Geometry: final body of the model. Coordinates: model frame, mm. A direction names the side the tool comes from. Give positions to 0.01 mm unless a question says otherwise; leave off trailing zeros. Order: outer loops, then holes, each group sorted by start corner. A loop starts at its lowest first (then second) coordinate and runs counter-clockwise, first axis right, second up. Notation, with made-up numbers: (-17.5, -39) - (3.5, -39) arc R25 ccw to (3.5, -26) - close; hole circle Ø1 at (-6.5, -3). An arc over 180 degrees is marked (long way). Use one line per item in the form item = value.
from build123d import *

# Parameters (mm, degrees)
SKETCH_1_R          = 25
EXTRUDE_1_DEPTH     = 4
SKETCH_4_R          = 2.05
CUT_EXTRUDE_1_DEPTH = 10
SKETCH_5_R          = 4.05
SKETCH_5_R_2        = 2.05
CUT_EXTRUDE_2_DEPTH = 1
SKETCH_6_R          = 25
SKETCH_6_R_2        = 20
CUT_EXTRUDE_3_DEPTH = 0.5


with BuildPart() as part:
    # 草图1 → 凸台-拉伸1 (new body)
    with BuildSketch(Plane.XY):
        Circle(SKETCH_1_R)
    extrude(amount=EXTRUDE_1_DEPTH)

    # 草图4 → 切除-拉伸1 (cut)
    with BuildSketch(Plane(origin=(0, 0, 0), x_dir=(-1, 0, 0), z_dir=(0, 0, -1))):
        with Locations((-10.392304845, -6)):
            Circle(SKETCH_4_R)
        with Locations((-10.392304845, 6)):
            Circle(SKETCH_4_R)
        with Locations((0, 12)):
            Circle(SKETCH_4_R)
        with Locations((10.392304845, 6)):
            Circle(SKETCH_4_R)
        with Locations((10.392304845, -6)):
            Circle(SKETCH_4_R)
        with Locations((0, -12)):
            Circle(SKETCH_4_R)
    extrude(amount=-CUT_EXTRUDE_1_DEPTH, mode=Mode.SUBTRACT)

    # 草图5 → 切除-拉伸2 (cut)
    with BuildSketch(Plane.XY.offset(4)):
        with Locations((-10.392304845, 6)):
            Circle(SKETCH_5_R)
        with Locations((-10.392304845, 6)):
            Circle(SKETCH_5_R_2, mode=Mode.SUBTRACT)
        with Locations((-10.392304845, -6)):
            Circle(SKETCH_5_R)
        with Locations((-10.392304845, -6)):
            Circle(SKETCH_5_R_2, mode=Mode.SUBTRACT)
        with Locations((0, -12)):
            Circle(SKETCH_5_R)
        with Locations((0, -12)):
            Circle(SKETCH_5_R_2, mode=Mode.SUBTRACT)
        with Locations((10.392304845, -6)):
            Circle(SKETCH_5_R)
        with Locations((10.392304845, -6)):
            Circle(SKETCH_5_R_2, mode=Mode.SUBTRACT)
        with Locations((10.392304845, 6)):
            Circle(SKETCH_5_R)
        with Locations((10.392304845, 6)):
            Circle(SKETCH_5_R_2, mode=Mode.SUBTRACT)
        with Locations((0, 12)):
            Circle(SKETCH_5_R)
        with Locations((0, 12)):
            Circle(SKETCH_5_R_2, mode=Mode.SUBTRACT)
    extrude(amount=-CUT_EXTRUDE_2_DEPTH, mode=Mode.SUBTRACT)

    # 草图6 → 切除-拉伸3 (cut)
    with BuildSketch(Plane(origin=(0, 0, 0), x_dir=(-1, 0, 0), z_dir=(0, 0, -1))):
        Circle(SKETCH_6_R)
        Circle(SKETCH_6_R_2, mode=Mode.SUBTRACT)
    extrude(amount=-CUT_EXTRUDE_3_DEPTH, mode=Mode.SUBTRACT)


solid = part.part
(1) Ray query, line 1 along Y through (x, z) = (0, 3.6); line 2 along X through (y, z) = (6, 2.3); line 3 along X through (y, z) = (-7, 0.2) (3 decimals). Return the intervals inside material, ascending.
Computed values:
line_1 = -25 to -16.05, -7.95 to 7.95, 16.05 to 25
line_2 = -24.27 to -12.44, -8.34 to 8.34, 12.44 to 24.27
line_3 = -18.735 to -12.182, -8.603 to 8.603, 12.182 to 18.735
(2) Cut plane D-D on y = -12. Output: boundary loops of the cut face in (x, z), plus the area to 3 significant figures.
Computed values:
outline = (-21.93, 0.5) - (-16, 0.5) - (-16, 0) - (-2.05, 0) - (-2.05, 3) - (-4.05, 3) - (-4.05, 4) - (-21.93, 4) - close; (2.05, 0) - (16, 0) - (16, 0.5) - (21.93, 0.5) - (21.93, 4) - (4.05, 4) - (4.05, 3) - (2.05, 3) - close
area = 149 mm²
(3) Cut plane C-C on y = -6. Output: boundary loops of the cut face in (x, z).
Computed values:
outline = (-24.27, 0.5) - (-19.08, 0.5) - (-19.08, 0) - (-12.44, 0) - (-12.44, 3) - (-14.44, 3) - (-14.44, 4) - (-24.27, 4) - close; (-8.34, 0) - (8.34, 0) - (8.34, 3) - (6.34, 3) - (6.34, 4) - (-6.34, 4) - (-6.34, 3) - (-8.34, 3) - close; (12.44, 0) - (19.08, 0) - (19.08, 0.5) - (24.27, 0.5) - (24.27, 4) - (14.44, 4) - (14.44, 3) - (12.44, 3) - close
(4) Reachability of faces 1 (the face through (-9, -8, 3)), 2 (the face through (4.336, -19.524, 0.246)), 3 (the face through (-8.344, 6.09, 1.479)) from +Z, -Z, +X, -X, +Y, -Y: full face, straight path, thin tool, end or side. Return the list, or none.
Computed values:
face_1 = +Z
face_2 = -Z
face_3 = +Z, -Z
(5) Cut plane A-A on z = 1.35. Output: boundary loops of the cut face in (x, y).
Computed values:
outline = circle Ø50 at (0, 0); hole circle Ø4.1 at (-10.39, -6); hole circle Ø4.1 at (-10.39, 6); hole circle Ø4.1 at (0, -12); hole circle Ø4.1 at (0, 12); hole circle Ø4.1 at (10.39, -6); hole circle Ø4.1 at (10.39, 6)
(6) Pull-direction query (X, two-part tool) for faces 4 (the face through (-8.344, -5.91, 1.479)), 5 (the face through (-0.878, 8.046, 3.507)), 6 (the face through (23.846, 7.509, 2.226)), 7 (the face through (11, 17, 0.5)); classes: released by +X, released by -X, zero draft, split by the parting line, or undercut.
Computed values:
face_4 = undercut
face_5 = undercut
face_6 = split by the parting line
face_7 = zero draft
(7) Contact query for flat-ended pins moving along their axis: pin 1 Ø13 at (x, y) = (-10.39, 6) entering from -Z; pin 2 Ø6.5 at (x, y) = (10.39, -6) entering from +Z; pin 3 Ø1.5 at (x, z) = (-4.5, 2.5) entering from -Y. Output: stop coordinate, or through.
Computed values:
pin_1 = 0
pin_2 = 3
pin_3 = -24.72
(8) Cut plane B-B on x = 0. Output: boundary loops of the cut face in (y, z).
Computed values:
outline = (-25, 0.5) - (-20, 0.5) - (-20, 0) - (-14.05, 0) - (-14.05, 3) - (-16.05, 3) - (-16.05, 4) - (-25, 4) - close; (-9.95, 0) - (9.95, 0) - (9.95, 3) - (7.95, 3) - (7.95, 4) - (-7.95, 4) - (-7.95, 3) - (-9.95, 3) - close; (14.05, 0) - (20, 0) - (20, 0.5) - (25, 0.5) - (25, 4) - (16.05, 4) - (16.05, 3) - (14.05, 3) - close
